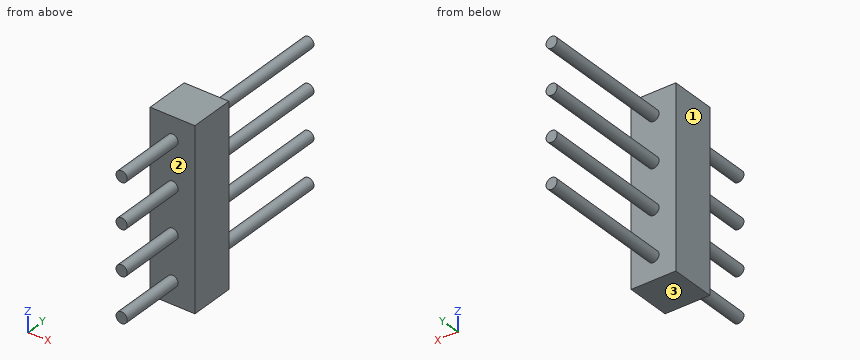
Autodesk Inventor part; units mm, degrees
ref_plane "YZ Plane" through (0, 0, 0) normal (1, 0, 0) x (0, 1, 0)
ref_plane "XZ Plane" through (0, 0, 0) normal (0, 1, 0) x (-1, 0, 0)
ref_plane "XY Plane" through (0, 0, 0) normal (0, 0, 1) x (1, 0, 0)
sketch "Sketch1" plane through (0, 0, 0) normal (0, 1, 0) x (-1, 0, 0)
  line L0 (-0.7674, 1.6667) -> (1.2326, 1.6667)
  line L1 (1.2326, 1.6667) -> (1.2326, -6.3333)
  line L2 (1.2326, -6.3333) -> (-0.7674, -6.3333)
  line L3 (-0.7674, -6.3333) -> (-0.7674, 1.6667)
  point P0 (0, 0)
  dimension "d0" = 2
  dimension "d1" = 8
extrude "Extrusion1" add sketch "Sketch1" along normal blind 2
sketch "Sketch2" plane through (0, 2, 0) normal (0, 1, 0) x (1, 0, 0)
  line L0 (0.7674, 6.3333) -> (-1.2326, 6.3333)
  circle A0 centre (-0.2326, 5.3333) radius 0.25
  point P0 (0, 0)
  dimension "d4" = 1
  dimension "d5" = 0.5
extrude "Extrusion2" add sketch "Sketch2" along normal blind 6 and the other way blind 5
pattern_linear "Rectangular Pattern1" count 4 spacing 2 along (0, 0, 1) of "Extrusion2"
properties part number "2mm4PosHeader"
Source: CAD feature listing. Evaluate the final solid. Frame: model axes, mm. Face numbers are marked on the shaded views. Give positions to 0.01 mm unless a question says otherwise; leave off trailing zeros. Write each loop counter-clockwise with the first axis right and the second up, starting at its lowest first coordinate (ties: lowest second). Pieces come first, ordered by that corner, then holes. Notation, with made-up numbers: (-38, 28.25) - (-27, 28.25) arc R19 cw to (-27, 63.25) - close; hole circle Ø10 at (36.25, -0.75). An arc over 180 degrees is marked (long way). Write item = value, one per line. Start each with the question number.
Q1. Cut plane C-C, the plane x = 0.5. Return loops of the section in (y, z), then the cut area to 3 significant figures.
Q2. Cut plane A-A, the plane z = -0.5. Return loops of the section in (x, y), then the cut area to 3 significant figures.
Q3. Cut plane B-B, the plane y = -1.25. Return loops of the section in (x, z).
Q4. Material intervals for probe 1 along Z at (x, y) = (-0.2, -0.75); probe 2 along Y at (x, z) = (-1.1, -1.75); probe 3 along Z at (x, y) = (-0.4, -1.25), sorted ascending.
Q5. Draft query along Z for the marked faces 1, 2 and 3. Return one class per face: +Z half, -Z half, draft (parallel to the pull), parting line (faces both ways), or undercut.
Q6. Pin query (flat end, axial travel): pin 1 Ø2 at (y, z) = (3.5, 0) entering from +X. Return the tip coordinate at first contact, or that it passes through.
Computed values:
q1.outline = (0, -6.33) - (2, -6.33) - (2, 1.67) - (0, 1.67) - close
q1.area = 16.0 mm²
q2.outline = (-1.23, 0) - (0.77, 0) - (0.77, 2) - (-1.23, 2) - close
q2.area = 4.00 mm²
q3.outline = circle Ø0.5 at (-0.23, -5.33); circle Ø0.5 at (-0.23, -3.33); circle Ø0.5 at (-0.23, -1.33); circle Ø0.5 at (-0.23, 0.67)
q4.probe_1 = -5.58 to -5.09, -3.58 to -3.09, -1.58 to -1.09, 0.42 to 0.91
q4.probe_2 = 0 to 2
q4.probe_3 = -5.52 to -5.15, -3.52 to -3.15, -1.52 to -1.15, 0.48 to 0.85
q5.face_1 = draft
q5.face_2 = undercut
q5.face_3 = -Z half
q6.pin_1 = 0.02
